Autodesk Inventor part; units mm, degrees
ref_plane "YZ Plane" through (0, 0, 0) normal (1, 0, 0) x (0, 1, 0)
ref_plane "XZ Plane" through (0, 0, 0) normal (0, 1, 0) x (-1, 0, 0)
ref_plane "XY Plane" through (0, 0, 0) normal (0, 0, 1) x (1, 0, 0)
sketch "Sketch1" plane through (0, 0, 0) normal (0, 1, 0) x (-1, 0, 0)
  line L0 (-7, 0) -> (-7, -45)
  line L1 (-7, 0) -> (-7, 45)
  line L2 (-7, 45) -> (7, 45)
  line L3 (7, 45) -> (7, -45)
  circle A0 centre (0, -38) radius 4
  line L4 (7, -45) -> (-7, -45)
  point P0 (0, 0)
  dimension "d4" = 45
  dimension "d5" = 45
  dimension "d6" = 14
  dimension "d7" = 90
  dimension "d8" = 8
  dimension "d9" = 7
extrude "Extrusion1" add sketch "Sketch1" along normal blind 6
fillet "Fillet1" radius 7 2 edges at (7, 3, -45) (-7, 3, -45)
sketch "Sketch2" plane through (0, 6, 0) normal (0, 1, 0) x (1, 0, 0)
  line L0 (-7, 38) -> (-7, -45)
  line L1 (-7, 30) -> (7, 30)
  line L2 (7, -45) -> (7, 38)
  arc A0 (7, 38) -> (-7, 38) centre (0, 38) ccw
  line L3 (-7, 30) -> (-7, -45)
  line L4 (-7, -45) -> (7, -45)
  line L5 (-7, -45) -> (7, -45)
  line L6 (7, -45) -> (7, 30)
  point P0 (0, 0)
  point P1 (0, 30)
  point P2 (0, 45)
  dimension "d13" = 15
extrude "Extrusion2" add sketch "Sketch2" along normal blind 8 contours L1 L2 L4 L0
sketch "Sketch3" plane through (0, 14, 0) normal (0, 1, 0) x (1, 0, 0)
  line L0 (-7, -45) -> (7, -45)
  line L1 (-7, -45) -> (-7, 45)
  line L2 (-7, 38) -> (-7, -45)
  line L3 (-7, 45) -> (7, 45)
  line L4 (7, -45) -> (7, 38)
  line L5 (7, 45) -> (7, -45)
  line L6 (7, -45) -> (-7, -45)
  circle A0 centre (0, 38) radius 4
  point P0 (0, 0)
  dimension "d16" = 90
  dimension "d17" = 8
  dimension "d18" = 7
extrude "Extrusion3" add sketch "Sketch3" along normal blind 6
fillet "Fillet2" radius 7 2 edges at (7, 17, -45) (-7, 17, -45)
draft "FaceDraft1" angle 3 pull direction (0, 1, 0) faces at (2.3333, 13.3333, 45) fixed edges at (0, 0, 45)
chamfer "Chamfer1" distance 0.02 angle 45 3 edges at (7, 20, 2.9759) (4.9498, 20, -42.9498) (-7, 20, 2.9759)
chamfer "Chamfer2" distance 0.02 angle 45 3 edges at (7, 0, 3.5) (4.9498, 0, -42.9498) (-7, 0, 3.4999)
chamfer "Chamfer3" distance 0.02 angle 45 3 edges at (6.98, 20, 2.9759) (4.9356, 20, -42.9356) (-6.98, 20, 2.9759)
chamfer "Chamfer4" distance 0.02 angle 45 3 edges at (-7, 0.02, 3.4994) (4.9498, 0.02, -42.9498) (7, 0.02, 3.4994)
properties part number "Schneidstempel"
Can you work these out from the model? Positions are in its coordinate system, mm. A direction names the side the tool comes from. Coordinates: 2 decimals unless noted, no trailing zeros. Answer as a JSON object with one key per item and string values. Group by question number.
Q1. Will these pins go through, and if not, where does the flat tip stop? P1, Ø6, axis at x = 0, y = 13, coming from the -Z side; P2, Ø3, axis at x = 3, y = 10, coming from the -Z side.
Q2. We'd pull the mould along Y, two halves only. Please class faces 1 (the face through (-4.9, 17, -43)), 2 (the face through (0, 20, -1)), 3 (the face through (0, 0, 1)), 4 (the face through (-2, 14, -34)): +Y half, -Y half, draft (parallel to the pull), parting line (faces both ways), or undercut.
Q3. On a 3-axis mill with a long thin cutter (end or side, diameter ignored), from which of +Z, -Z, +X, -X, +Y, -Y can I reach the whole of each face in a straight line? I mean faces 5 (the face through (0.521, 2.958, -41.966)), 6 (the face through (2, 6, -34)). Say none if no direction works.
Q4. I need wall thicknesses on line 1 (Y direction, x = -6, z = -41); line 2 (X direction, y = 17.1, z = -38); line 3 (Z direction, x = 0, y = 17.2). Which ranges of each line are inside material? Lowest first, please. Write a range as from..to.
Determined:
{
 "1": {"P1": "stops at z = -45", "P2": "stops at z = -30"},
 "2": {"face 1": "draft", "face 2": "+Y half", "face 3": "-Y half", "face 4": "undercut"},
 "3": {"face 5": "+Y, -Y", "face 6": "-Z, +X, -X"},
 "4": {"line 1": "y = 0..6, 14..20", "line 2": "x = -7..-4, 4..7", "line 3": "z = -45..-42, -34..44.1"}
}
